Can you work these out from the drawing? Everything is in mm from the part's minimum corner. A direction names the side the tool comes from. Round coordinates to 2 decimals unless told otherwise and drop trailing zeros. Loops run counter-clockwise (first coordinate to the right, second up) from the corner with the lowest first, then second, coordinate; pieces in that order, holes last. Notation, with made-up numbers: (-25.75, 2.25) - (-2.75, 2.25) arc R31 ccw to (-2.75, 41.25) - close; hole circle Ø1 at (27, 79). An arc over 180 degrees is marked (long way). Return JSON: item names as keys, results as strings. Group by question number.
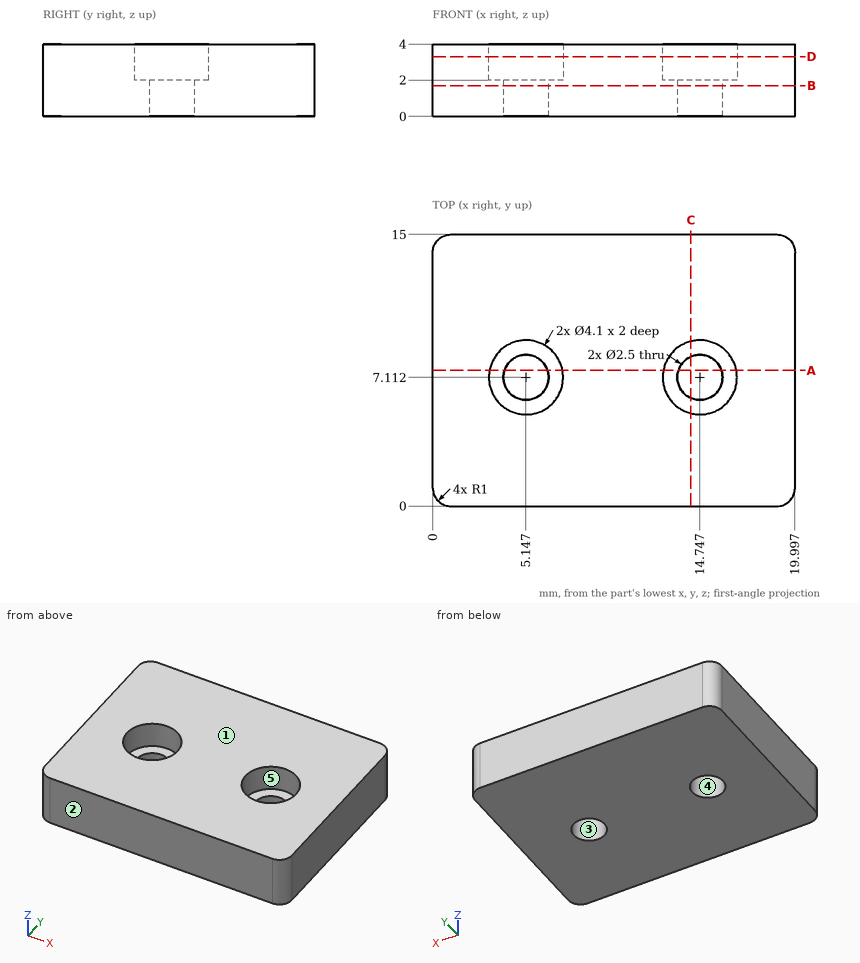
Q1. Imagine slicing it at C-C, the plane x = 14.25. List the corners of the cut face in (y, z) for me (1 decimal).
Q2. Please list where these lines run through material, in increasing order: line 1 (Y direction, x = 5.25, z = 2.35) (1 decimal); line 2 (X direction, y = 7.5, z = 1.5) (1 decimal); line 3 (X direction, y = 6, z = 0.8) (1 decimal).
Q3. Imagine slicing it at D-D, the plane z = 3.3. List the corners of the cut face in (x, y) for me, and give its area (3 significant figures).
Q4. Will these pins go through, and if not, where does the flat tip stop? pin 1 Ø2 at (x, y) = (5.15, 7.11) entering from -Z; pin 2 Ø4 at (x, y) = (14.75, 7.11) entering from +Z.
Q5. For the marked faces 4 and 5, which set-ups out of +Z, -Z, +X, -X, +Y, -Y let a thin tool reach every point of the face, with its end or its side?
Q6. If we mould it in two halves opening along Y, with no side actions, what happens to the marked faces 1, 2 and 3? For each: +Y half, -Y half, draft (parallel to the pull), parting line (faces both ways), or undercut.
Q7. Imagine slicing it at A-A, the plane y = 7.5. List the corners of the cut face in (x, z) for me (1 decimal).
Q8. Imagine slicing it at B-B, the plane z = 1.7. List the corners of the cut face in (x, y) for me, and give its area (3 significant figures).
Output values:
{
 "1": {"outline": "(0, 0) - (6, 0) - (6, 2) - (5.1, 2) - (5.1, 4) - (0, 4) - close; (8.3, 0) - (15, 0) - (15, 4) - (9.1, 4) - (9.1, 2) - (8.3, 2) - close"},
 "2": {"line 1": "y = 0 to 5.1, 9.2 to 15", "line 2": "x = 0 to 4, 6.3 to 13.6, 15.9 to 20", "line 3": "x = 0 to 4.6, 5.7 to 14.2, 15.3 to 20"},
 "3": {"outline": "(0, 1) arc R1 ccw to (1, 0) - (19, 0) arc R1 ccw to (20, 1) - (20, 14) arc R1 ccw to (19, 15) - (1, 15) arc R1 ccw to (0, 14) - close; hole circle Ø4.1 at (5.15, 7.11); hole circle Ø4.1 at (14.75, 7.11)", "area": "273 mm^2"},
 "4": {"pin 1": "passes through", "pin 2": "stops at z = 2"},
 "5": {"face 4": "+Z, -Z", "face 5": "+Z"},
 "6": {"face 1": "draft", "face 2": "-Y half", "face 3": "undercut"},
 "7": {"outline": "(0, 0) - (4, 0) - (4, 2) - (3.1, 2) - (3.1, 4) - (0, 4) - close; (6.3, 0) - (13.6, 0) - (13.6, 2) - (12.7, 2) - (12.7, 4) - (7.2, 4) - (7.2, 2) - (6.3, 2) - close; (15.9, 0) - (20, 0) - (20, 4) - (16.8, 4) - (16.8, 2) - (15.9, 2) - close"},
 "8": {"outline": "(0, 1) arc R1 ccw to (1, 0) - (19, 0) arc R1 ccw to (20, 1) - (20, 14) arc R1 ccw to (19, 15) - (1, 15) arc R1 ccw to (0, 14) - close; hole circle Ø2.5 at (5.15, 7.11); hole circle Ø2.5 at (14.75, 7.11)", "area": "289 mm^2"}
}
